Geometry: see drawing. Coordinates: mm, zero at the bounding-box minimum. A direction names the side the tool comes from. Give positions to 0.01 mm unless a question says otherwise; leave off trailing zeros. Order: outer loops, then holes, each group sorted by start corner. A loop starts at its lowest first (then second) coordinate and runs counter-clockwise, first axis right, second up. Notation, with made-up numbers: M 29.5,7.5 L 67.5,7.5 A17 ccw 67.5,17.5 Z; hole C 82.5,-9.5 d4. An arc over 180 degrees is marked long. Write item = value, one per line. Start each with the question number.
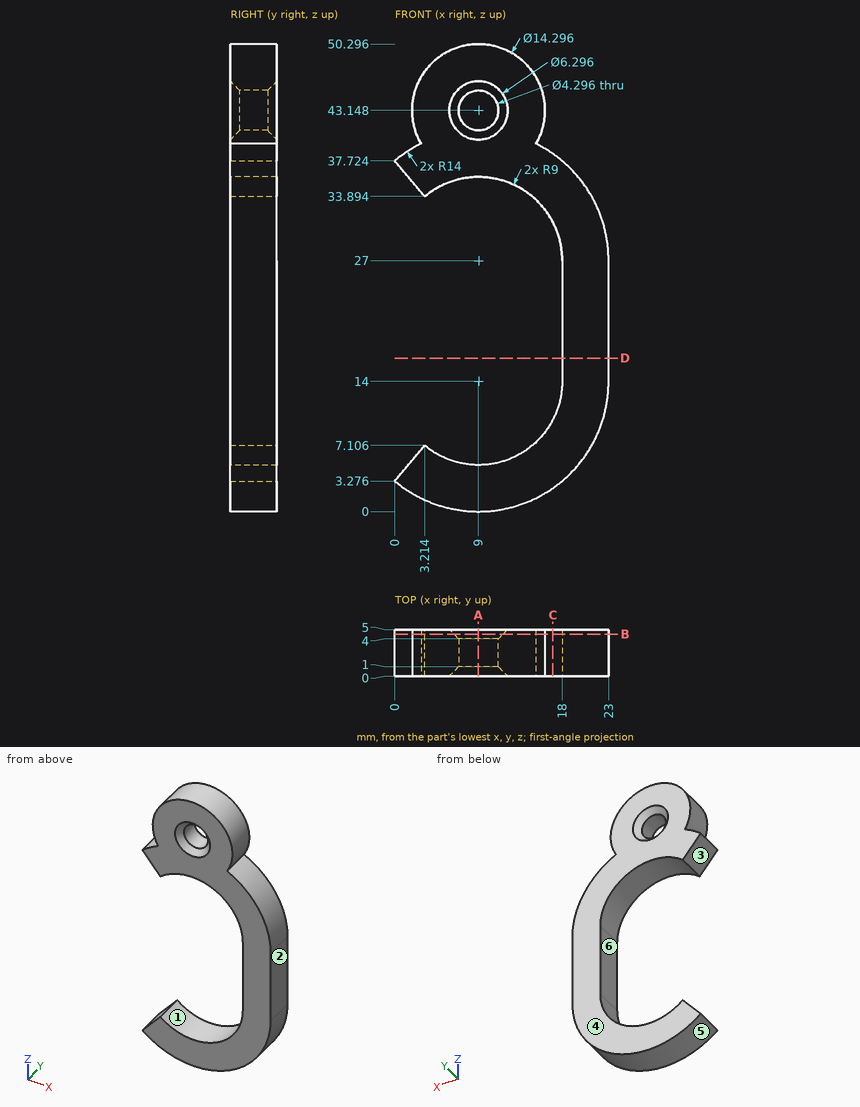
1) Cut plane A-A (x = 9). Return loops of the section in (y, z).
2) Cut plane B-B (y = 4.5). Return loops of the section in (x, z) (1 decimal), plus the area to 3 significant figures.
3) Pin query (flat end, axial travel): pin 1 Ø10 at (x, z) = (13.5, 43) entering from -Y; pin 2 Ø4 at (x, z) = (15.5, 20) entering from +Y; pin 3 Ø5.5 at (x, z) = (9, 43.15) entering from +Y (1 decimal); pin 4 Ø2 at (x, y) = (7, 1.5) entering from +Z. Return the tip coordinate at first contact, or that it passes through.
4) Cut plane C-C (x = 17). Return loops of the section in (y, z).
5) Draft query along Z for the marked faces 4, 5 and 6. Return one class per face: pulls with the +Z half, pulls with the -Z half, needs draft (parallel to the pull), parting line crosses it, or undercut.
6) Access query for the marked faces 1, 2 and 3. Directions: +Z, -Z, +X, -X, +Y, -Y. A direction counts if a zero-diameter tool reaches every point of the face in a straight line with its end or side. Return the directions, or none.
7) Cut plane D-D (z = 16.5). Return loops of the section in (x, y).
8) Ray query, L1, parallel to Z at x = 10.25, y = 3.2 (1 decimal); L2, parallel to Z at x = 13.75, y = 4.2 (1 decimal); L3, parallel to X at y = 3, z = 45 (1 decimal). Return the intervals inside material, ascending.
Reply:
q1.outline = M 0,0 L 5,0 L 5,5 L 0,5 Z; M 0,36 L 5,36 L 5,40 L 4,41 L 1,41 L 0,40 Z; M 0,46.3 L 1,45.3 L 4,45.3 L 5,46.3 L 5,50.3 L 0,50.3 Z
q2.outline = M 0,3.3 A14 ccw 23,14 L 23,27 A14 ccw 15.2,39.6 A7.1 ccw long 2.8,39.6 A14 ccw 0,37.7 L 3.2,33.9 A9 cw 18,27 L 18,14 A9 cw 3.2,7.1 Z; hole C 9,43.1 d5.3
q2.area = 421 mm²
q3.pin_1 = 0
q3.pin_2 = through
q3.pin_3 = 4.6
q3.pin_4 = 50.23
q4.outline = M 0,2.51 L 5,2.51 L 5,9.88 L 0,9.88 Z; M 0,31.12 L 5,31.12 L 5,38.49 L 0,38.49 Z
q5.face_4 = needs draft
q5.face_5 = pulls with the -Z half
q5.face_6 = undercut
q6.face_1 = +Y, -Y
q6.face_2 = +Z, -Z, +X, +Y, -Y
q6.face_3 = -X, +Y, -Y
q7.outline = M 18,0 L 23,0 L 23,5 L 18,5 Z
q8.L1 = 0.1 to 5.1, 35.9 to 41.4, 44.9 to 50.2
q8.L2 = 0.8 to 6.4, 34.6 to 48.5
q8.L3 = 2.1 to 7.9, 10.1 to 15.9
